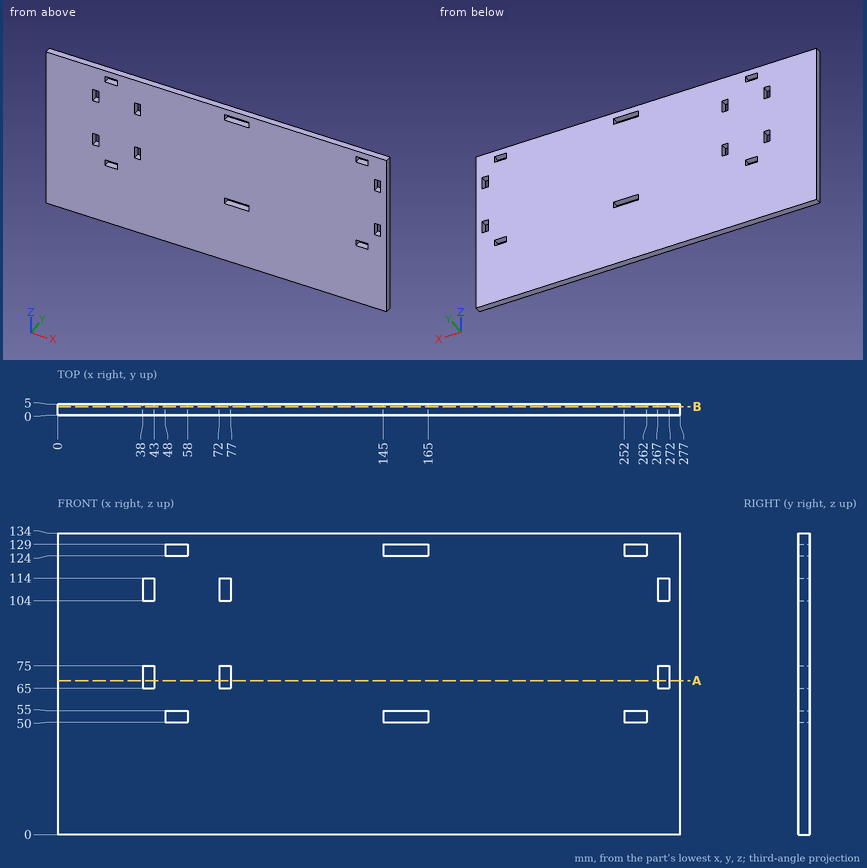
Source: three-view drawing plus pictorial views. Frame: mm from the lowest corner of the part. Round coordinates to 2 decimals unless told otherwise and drop trailing zeros. Loops run counter-clockwise (first coordinate to the right, second up) from the corner with the lowest first, then second, coordinate; pieces in that order, holes last. Notation, with made-up numbers: M -7,-7.75 L 2,-7.75 A25 ccw 2,8.25 Z; hole C 70,57.25 d9. An arc over 180 degrees is marked long. Answer as CSV lines item,"result". Start each with the question number.
(1) Section A-A, the plane z = 68.5. Output: boundary loops of the cut face in (x, y), plus the area to 3 significant figures.
(2) Section B-B, the plane y = 3.85. State how many separate pieces and enclosed holes the cut face has, plus the area to 3 significant figures.
(3) Line query: line 1 (X direction, y = 1.6, z = 127); line 2 (Z direction, x = 72.5, y = 1.7); line 3 (X direction, y = 0.5, z = 67). Output: solid intervals per line, ascending. Write a range as [from, to].
Values found:
1,outline,"M 0,0 L 38,0 L 38,5 L 0,5 Z; M 43,0 L 72,0 L 72,5 L 43,5 Z; M 77,0 L 267,0 L 267,5 L 77,5 Z; M 272,0 L 277,0 L 277,5 L 272,5 Z"
1,area,"1,310 mm²"
2,separate pieces,"1"
2,enclosed holes,"12"
2,area,"36,400 mm²"
3,line 1,"x = [0, 48], [58, 145], [165, 252], [262, 277]"
3,line 2,"z = [0, 65], [75, 104], [114, 134]"
3,line 3,"x = [0, 38], [43, 72], [77, 267], [272, 277]"
